Work out the finished part from the listing and answer in its coordinate system (mm). A direction names the side the tool comes from. Give positions to 0.01 mm unless a question says otherwise; leave off trailing zeros. Order: outer loops, then holes, each group sorted by start corner. A loop starts at its lowest first (then second) coordinate and runs counter-clockwise, first axis right, second up.
```python
from build123d import *

# Parameters (mm, degrees)
SKETCH1_W           = 16.5
SKETCH1_H           = 11.5
SKETCH1_W_2         = 10.5
SKETCH1_H_2         = 5.5
BOSS_EXTRUDE1_DEPTH = 17
CUT_EXTRUDE1_REACH  = 28.334
SKETCH2_R           = 2.5
SKETCH3_W           = 16.5
SKETCH3_H           = 11.5
BOSS_EXTRUDE2_DEPTH = 3
BOSS_EXTRUDE3_START = -11
SKETCH4_W           = 21.75
SKETCH4_H           = 11
BOSS_EXTRUDE3_DEPTH = 4
CHAMFER1_SIZE       = 5
CHAMFER2_SIZE       = 3
SKETCH5_R           = 1.1
SKETCH5_W           = 3
SKETCH5_H           = 2.684
BOSS_EXTRUDE4_DEPTH = 7
BOSS_EXTRUDE5_DEPTH = 11
CUT_EXTRUDE2_REACH  = 41.144
SKETCH7_W           = 10.5
SKETCH7_H           = 1.5
CUT_EXTRUDE3_REACH  = 38.011
SKETCH8_W           = 21.5
SKETCH8_H           = 19.176
SKETCH8_W_2         = 4
SKETCH8_H_2         = 11
SKETCH9_W           = 12
SKETCH9_H           = 4
BOSS_EXTRUDE6_DEPTH = 8.5
SKETCH10_W          = 18.65
SKETCH10_H          = 3.47
BOSS_EXTRUDE7_DEPTH = 6.35


with BuildPart() as part:
    # Sketch1 → Boss-Extrude1 (new body)
    with BuildSketch(Plane(origin=(0, 0, 0), x_dir=(1, 0, 0), z_dir=(0, 1, 0))):
        with Locations((8.25, 5.75)):
            Rectangle(SKETCH1_W, SKETCH1_H)
        with Locations((8.25, 5.75)):
            Rectangle(SKETCH1_W_2, SKETCH1_H_2, mode=Mode.SUBTRACT)
    extrude(amount=BOSS_EXTRUDE1_DEPTH)

    # Sketch2 → Cut-Extrude1 (cut, up to next)
    with BuildSketch(Plane(origin=(0, 0, -11.5), x_dir=(-1, 0, 0), z_dir=(0, 0, -1)), mode=Mode.PRIVATE) as cut_extrude1_sk1:
        with Locations((-8.25, 10.5)):
            Circle(SKETCH2_R)
    cut_extrude1_tool1 = extrude(cut_extrude1_sk1.sketch, amount=-CUT_EXTRUDE1_REACH, mode=Mode.PRIVATE) & part.part
    add(cut_extrude1_tool1.solids().sort_by_distance((8.25, 10.5, -11.5))[0], mode=Mode.SUBTRACT)

    # Sketch3 → Boss-Extrude2 (add)
    with BuildSketch(Plane(origin=(0, 17, 0), x_dir=(1, 0, 0), z_dir=(0, 1, 0))):
        with Locations((8.25, 5.75)):
            Rectangle(SKETCH3_W, SKETCH3_H)
    extrude(amount=BOSS_EXTRUDE2_DEPTH)

    # Sketch4 → Boss-Extrude3 (add)
    with BuildSketch(Plane(origin=(0, 20, 0), x_dir=(1, 0, 0), z_dir=(0, 1, 0)).offset(BOSS_EXTRUDE3_START)):
        with Locations((-10.875, -2.176)):
            Rectangle(SKETCH4_W, SKETCH4_H)
    extrude(amount=BOSS_EXTRUDE3_DEPTH)

    # Chamfer1
    chamfer1_edges = [part.edges().sort_by_distance(p)[0] for p in [
        (0, 11, 0),
        (0, 11, -3.324),
    ]]
    chamfer(chamfer1_edges, length=CHAMFER1_SIZE)

    # Chamfer2
    chamfer2_edges = [part.edges().sort_by_distance(p)[0] for p in [
        (0, 13, -4.162),
        (0, 9, -4.162),
        (2.5, 13, 0),
        (2.5, 9, 0),
    ]]
    chamfer(chamfer2_edges, length=CHAMFER2_SIZE)

    # Sketch5 → Boss-Extrude4 (add)
    with BuildSketch(Plane(origin=(0, 13, 0), x_dir=(1, 0, 0), z_dir=(0, 1, 0))):
        with Locations(Location((-19.15, -2.46, 0), (0, 0, 270))):
            Circle(SKETCH5_R)
        with Locations(Location((-9.5, -2.46, 0), (0, 0, 270))):
            Circle(SKETCH5_R)
        with Locations((-19.15, 1.982)):
            Rectangle(SKETCH5_W, SKETCH5_H)
        with Locations((-9.5, 1.982)):
            Rectangle(SKETCH5_W, SKETCH5_H)
    extrude(amount=BOSS_EXTRUDE4_DEPTH)

    # Sketch6 → Boss-Extrude5 (add)
    with BuildSketch(Plane.XY.offset(7.676)):
        Polygon((-21.75, 13), (-24.65, 13), (-24.65, 20), (-27.65, 20), (-27.65, 9), (-21.75, 9), align=None)
    extrude(amount=-BOSS_EXTRUDE5_DEPTH)

    # Sketch7 → Cut-Extrude2 (cut, up to next)
    with BuildSketch(Plane(origin=(0, 0, -11.5), x_dir=(-1, 0, 0), z_dir=(0, 0, -1)), mode=Mode.PRIVATE) as cut_extrude2_sk1:
        with Locations((-8.25, 16.25)):
            Rectangle(SKETCH7_W, SKETCH7_H)
    cut_extrude2_tool1 = extrude(cut_extrude2_sk1.sketch, amount=-CUT_EXTRUDE2_REACH, mode=Mode.PRIVATE) & part.part
    add(cut_extrude2_tool1.solids().sort_by_distance((8.25, 16.25, -11.5))[0], mode=Mode.SUBTRACT)

    # Sketch8 → Cut-Extrude3 (cut, up to next)
    with BuildSketch(Plane(origin=(0, 20, 0), x_dir=(1, 0, 0), z_dir=(0, 1, 0)), mode=Mode.PRIVATE) as cut_extrude3_sk1:
        with Locations((5.75, 1.912)):
            Rectangle(SKETCH8_W, SKETCH8_H)
    cut_extrude3_tool1 = extrude(cut_extrude3_sk1.sketch, amount=-CUT_EXTRUDE3_REACH, mode=Mode.PRIVATE) & part.part
    # Sketch8 → Cut-Extrude3 (cut, up to next)
    with BuildSketch(Plane(origin=(0, 20, 0), x_dir=(1, 0, 0), z_dir=(0, 1, 0)), mode=Mode.PRIVATE) as cut_extrude3_sk2:
        with Locations((-25.65, -2.176)):
            Rectangle(SKETCH8_W_2, SKETCH8_H_2)
    cut_extrude3_tool2 = extrude(cut_extrude3_sk2.sketch, amount=-CUT_EXTRUDE3_REACH, mode=Mode.PRIVATE) & part.part
    add(cut_extrude3_tool1.solids().sort_by_distance((5.75, 20, -1.912))[0], mode=Mode.SUBTRACT)
    add(cut_extrude3_tool2.solids().sort_by_distance((-25.65, 20, 2.176))[0], mode=Mode.SUBTRACT)

    # Sketch9 → Boss-Extrude6 (add)
    with BuildSketch(Plane.XZ.offset(-9)):
        with Locations((-14.325, 4.978)):
            Rectangle(SKETCH9_W, SKETCH9_H)
    extrude(amount=BOSS_EXTRUDE6_DEPTH)

    # Sketch10 → Boss-Extrude7 (add)
    with BuildSketch(Plane.XZ.offset(-9)):
        with Locations((-14.325, -1.589)):
            Rectangle(SKETCH10_W, SKETCH10_H)
    extrude(amount=BOSS_EXTRUDE7_DEPTH)


solid = part.part
```
1. Straight lines are drawn through the part: probe 1 along Z at (x, y) = (-18.25, 7); probe 2 along Y at (x, z) = (-17.25, 1); probe 3 along Y at (x, z) = (-12.5, 6). For each, find the intervals that lie inside material, in ascending order.
Findings below:
probe 1: z = -3.32 to 0.15, 2.98 to 6.98
probe 2: y = 9 to 13
probe 3: y = 0.5 to 13
2. Which of the six approach directions +Z, -Z, +X, -X, +Y, -Y give full straight-line access (tool end or side, diameter ignored) to faces 1 (the face through (-20.325, 5, 5)), 2 (the face through (-8.325, 5, 5)), 3 (the face through (-19, 16, -0.64))?
Findings below:
face 1: +Z, -X, -Y
face 2: +Z, +X, -Y
face 3: +X, -X, +Y
3. The part is cut by section D-D (x = -15.5). Write down the section's boundary in (y, z).
Findings below:
outline: (0.5, 2.98) - (9, 2.98) - (9, 0.15) - (2.65, 0.15) - (2.65, -3.32) - (13, -3.32) - (13, 7.68) - (9, 7.68) - (9, 6.98) - (0.5, 6.98) - close
4. Given P1, Ø0.8, axis at y = 15, z = -1.5, coming from the -X side; P2, Ø2.5, axis at x = -11.5, y = 3.5, coming from the +Z side; P3, Ø3, axis at y = 18, z = -2, coming from the +X side, each flat-ended and moving along its own axis, determine where each tip first touches the part or whether it passes through.
Findings below:
P1: stops at x = -20.65
P2: stops at z = 6.98
P3: stops at x = -8
5. The part is cut by section C-C (z = 2.46). Write down the section's boundary in (x, y).
Findings below:
outline: (-23.65, 9) - (-5, 9) - (-5, 13) - (-8.4, 13) - (-8.4, 20) - (-10.6, 20) - (-10.6, 13) - (-18.05, 13) - (-18.05, 20) - (-20.25, 20) - (-20.25, 13) - (-23.65, 13) - close
6. The mould has two halves that part along X. Classify faces 4 (the face through (-14, 13, 2)), 5 (the face through (-10, 20, -2)), 6 (the face through (-8, 16, -2)): pulls with the +X half, pulls with the -X half, needs draft (parallel to the pull), parting line crosses it, or undercut.
Findings below:
face 4: undercut
face 5: needs draft
face 6: pulls with the +X half
7. The part is cut by section A-A (y = 3.25). Write down the section's boundary in (x, z) (3 decimals).
Findings below:
outline: (-23.65, -3.324) - (-5, -3.324) - (-5, 0.146) - (-23.65, 0.146) - close; (-20.325, 2.978) - (-8.325, 2.978) - (-8.325, 6.978) - (-20.325, 6.978) - close
8. The part is cut by section B-B (y = 16). Write down the section's boundary in (x, z).
Findings below:
outline: (-20.65, -3.32) - (-17.65, -3.32) - (-17.65, -0.64) - (-20.65, -0.64) - close; circle Ø2.2 at (-19.15, 2.46); (-11, -3.32) - (-8, -3.32) - (-8, -0.64) - (-11, -0.64) - close; circle Ø2.2 at (-9.5, 2.46)
